For this review, take the finished solid that the model builds, in its own axes (mm). Face numbers are marked on the shaded views. A direction names the side the tool comes from. Coordinates: 2 decimals unless noted, no trailing zeros. Order: outer loops, then holes, each group sorted by start corner. A loop starts at its lowest first (then second) coordinate and runs counter-clockwise, first axis right, second up. Notation, with made-up numbers: (-17.5, -18.75) -> (-7.5, -18.75) arc R6 ccw to (-7.5, -9.75) -> close; hole circle Ø5 at (-9, 89.5). An arc over 180 degrees is marked (long way). Answer as a JSON object with one key per item and string values. Group by question number.
1) Add section C-C, the plane y = 2.1. Write out the cut boundary in (x, z), then the cut area to 3 significant figures.
2) Add section D-D, the plane z = 4.5. Count the separate pieces of the cut face and the enclosed holes in it, then the cut area to 3 significant figures.
3) Machinability: for the marked faces 1 and 2, which of the approach directions +Z, -Z, +X, -X, +Y, -Y give a long, thin tool a straight path to every point of the face, cutting with its end or side? Answer none if there is none.
4) Add section B-B, the plane x = -18. Write out the cut boundary in (y, z).
5) Add section A-A, the plane y = 5.6. Write out the cut boundary in (x, z).
6) Draft analysis for pull direction Z (two halves, no side actions). For the marked faces 3, 4 and 5, state which applies: +Z half, -Z half, draft (parallel to the pull), parting line (faces both ways), or undercut.
7) For pin 1 (3.5 mm diameter, centred on x = 18, z = 4.5, fed in from +Y); pin 2 (1.7 mm diameter, centred on x = 21, z = 4, fed in from +Y); pin 3 (1.9 mm diameter, centred on x = -12.5, z = 4.5, fed in from +Y), all flat-tipped, find the tip position at first contact; note any pin that passes through.
8) Wall thickness on L1, parallel to Z at x = 12.5, y = 0.25; L2, parallel to Z at x = -12.5, y = 3.05; L3, parallel to X at y = 0.4, z = 6.75: over which ranges is each line inside the solid? List them lowest first.
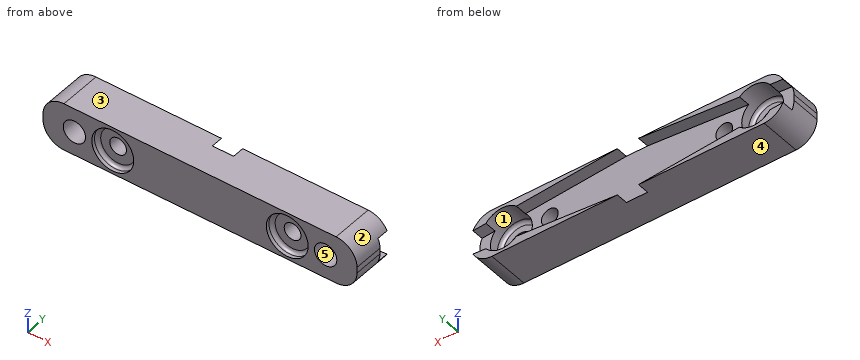
from build123d import *

# Parameters (mm, degrees)
SKETCH_2_R               = 1.2
SKETCH_2_R_2             = 1.6
EXTRUDE_2_DEPTH          = 6
SKETCH_3_R               = 3
CUT_EXTRUDE_1_DEPTH      = 1
FILLET_2_R               = 3
CUT_EXTRUDE_2_DEPTH      = 1.7
SKETCH_5_R               = 3
CUT_EXTRUDE_3_DEPTH      = 2.7
CUT_EXTRUDE_3_DEPTH_BACK = 1.8
FILLET_3_R               = 0.5


with BuildPart() as part:
    # 草图2 → 凸台-拉伸2 (new body)
    with BuildSketch(Plane(origin=(0, 0, 4.5), x_dir=(1, 0, 0), z_dir=(0, 1, 0))):
        Polygon((22.5, -3.42139756), (22.5, 3.421397553), (3.906515802, 3.421397553), (-3.906515802, 3.421397553), (-22.5, 3.421397553), (-22.5, -3.42139756), (-3.906515802, -3.42139756), (3.906515802, -3.42139756), align=None)
        with Locations((-12.5, -3e-09)):
            Circle(SKETCH_2_R, mode=Mode.SUBTRACT)
        with Locations((12.5, -3e-09)):
            Circle(SKETCH_2_R, mode=Mode.SUBTRACT)
        with Locations((-18, -3e-09)):
            Circle(SKETCH_2_R_2, mode=Mode.SUBTRACT)
        with Locations((18, -3e-09)):
            Circle(SKETCH_2_R_2, mode=Mode.SUBTRACT)
    extrude(amount=EXTRUDE_2_DEPTH)

    # 草图3 → 切除-拉伸1 (cut)
    with BuildSketch(Plane(origin=(0, 0, 0), x_dir=(-1, 0, 0), z_dir=(0, -1, 0))):
        with Locations((-12.5, -4.500000003)):
            Circle(SKETCH_3_R)
        with Locations((12.5, -4.500000003)):
            Circle(SKETCH_3_R)
    extrude(amount=-CUT_EXTRUDE_1_DEPTH, mode=Mode.SUBTRACT)

    # 圆角2
    fillet_2_edges = [part.edges().sort_by_distance(p)[0] for p in [
        (22.5, 3, 1.078602447),
        (22.5, 3, 7.92139756),
        (-22.5, 3, 7.92139756),
        (-22.5, 3, 1.078602447),
    ]]
    fillet(fillet_2_edges, radius=FILLET_2_R)

    # 草图4 → 切除-拉伸2 (cut)
    with BuildSketch(Plane(origin=(0, 6, 0), x_dir=(1, 0, 0), z_dir=(0, 1, 0))):
        Polygon((43.079074711, -4.500000003), (0, -8.046158962), (-43.079074711, -4.500000003), (0, -0.953841045), align=None)
    extrude(amount=-CUT_EXTRUDE_2_DEPTH, mode=Mode.SUBTRACT)

    # 草图5 → 切除-拉伸3 (cut, two sides)
    with BuildSketch(Plane(origin=(0, 4.3, 0), x_dir=(1, 0, 0), z_dir=(0, 1, 0))) as cut_extrude_3_sk:
        with Locations((-18, -4.500000003)):
            Circle(SKETCH_5_R)
        with Locations((18, -4.500000003)):
            Circle(SKETCH_5_R)
    extrude(amount=CUT_EXTRUDE_3_DEPTH, mode=Mode.SUBTRACT)
    extrude(cut_extrude_3_sk.sketch, amount=-CUT_EXTRUDE_3_DEPTH_BACK, mode=Mode.SUBTRACT)

    # 圆角3
    fillet_3_edges = [part.edges().sort_by_distance(p)[0] for p in [
        (-21, 2.5, 4.500000003),
        (15, 2.5, 4.500000003),
        (15.5, 1, 4.500000003),
        (-9.5, 1, 4.500000003),
    ]]
    fillet(fillet_3_edges, radius=FILLET_3_R)


solid = part.part
Output values:
{
 "1": {"outline": "(-22.5, 4.08) arc R3 ccw to (-19.5, 1.08) -> (19.5, 1.08) arc R3 ccw to (22.5, 4.08) -> (22.5, 4.92) arc R3 ccw to (19.5, 7.92) -> (-19.5, 7.92) arc R3 ccw to (-22.5, 4.92) -> close; hole circle Ø3.2 at (-18, 4.5); hole circle Ø2.4 at (-12.5, 4.5); hole circle Ø2.4 at (12.5, 4.5); hole circle Ø3.2 at (18, 4.5)", "area": "275 mm²"},
 "2": {"separate pieces": "5", "enclosed holes": "0", "area": "128 mm²"},
 "3": {"face 1": "+Y", "face 2": "+Z, +X, +Y, -Y"},
 "4": {"outline": "(0, 1.08) -> (6, 1.08) -> (6, 1.5) -> (3, 1.5) arc R0.5 cw to (2.5, 2) -> (2.5, 2.9) -> (0, 2.9) -> close; (0, 6.1) -> (2.5, 6.1) -> (2.5, 7) arc R0.5 cw to (3, 7.5) -> (6, 7.5) -> (6, 7.92) -> (0, 7.92) -> close"},
 "5": {"outline": "(-22.21, 2.78) arc R3 ccw to (-19.5, 1.08) -> (-1.52, 1.08) -> (-15.99, 2.27) arc R3 cw to (-20.34, 2.63) -> close; (-22.21, 6.22) -> (-20.34, 6.37) arc R3 cw to (-15.99, 6.73) -> (-1.52, 7.92) -> (-19.5, 7.92) arc R3 ccw to start; (1.52, 1.08) -> (19.5, 1.08) arc R3 ccw to (22.21, 2.78) -> (20.34, 2.63) arc R3 cw to (15.99, 2.27) -> close; (1.52, 7.92) -> (15.99, 6.73) arc R3 cw to (20.34, 6.37) -> (22.21, 6.22) arc R3 ccw to (19.5, 7.92) -> close"},
 "6": {"face 3": "+Z half", "face 4": "-Z half", "face 5": "undercut"},
 "7": {"pin 1": "stops at y = 2.5", "pin 2": "stops at y = 4.3", "pin 3": "passes through"},
 "8": {"L1": "z = 1.08 to 1.5, 7.5 to 7.92", "L2": "z = 1.08 to 3.3, 5.7 to 7.92", "L3": "x = -21.88 to -14.48, -10.52 to 10.52, 14.48 to 21.88"}
}
